Read the model definition and answer for the solid it produces. Units are mm, in the model's axes. A direction names the side the tool comes from. Give positions to 0.01 mm unless a question says otherwise; leave off trailing zeros. Loops run counter-clockwise (first coordinate to the right, second up) from the corner with the lowest first, then second, coordinate; pieces in that order, holes last. Notation, with made-up numbers: (19, -14) -> (78, -14) arc R17 ccw to (78, -2) -> close; hole circle Ø5 at (-3.75, 41). An arc over 180 degrees is marked (long way). Write each question's results on one line, items separated by ' | '. Start each with the question number.
Item 1: Each of these flat-tipped pins is pushed along its axis until it touches: P1, Ø0.7, axis at x = -4, y = -0.5, coming from the -Z side; P2, Ø5, axis at x = 0, z = 39, coming from the +Y side; P3, Ø3, axis at y = -2.5, z = 0.5, coming from the -X side. Where does it stop, or does it pass through?
Item 2: Determine the mould class of faces 1 (the flat face through (-0.1, 1.6, 35.7)), 2 (the flat face through (2, -2, -12)), 3 (the cylindrical face through (0, -2, 0)), 4 (the cylindrical face through (0, 0, 43)) for opening direction Z: +Z half, -Z half, draft (parallel to the pull), parting line (faces both ways), or undercut.
Item 3: Section B-B on x = 0 is taken. Write down the section's boundary in (y, z).
Item 4: Section C-C on z = 15 is taken. Write down the section's boundary in (x, y), and give its area (3 significant figures).
Item 5: Section A-A on y = 0 is taken. State how many separate pieces and enclosed holes the cut face has, and give its area (3 significant figures).
Item 6: Find the intervals of material crossed by line 1 (Z direction, x = 0, y = 1.5); line 2 (Y direction, x = 4, z = 38); line 3 (Z direction, x = -1.75, y = -0.75), in increasing order.
Item 7: Which of the six approach directions +Z, -Z, +X, -X, +Y, -Y give full straight-line access (tool end or side, diameter ignored) to faces 5 (the flat face through (-0.1, 1.6, -35.7)), 6 (the flat face through (-0.1, -1.6, -35.7)), 7 (the flat face through (2, -2, 12)), 8 (the flat face through (-0.1, -1.6, 35.7))?
```python
from build123d import *

# Parameters (mm, degrees)
SKETCH1_R                  = 2
SCREW_SECTION_DEPTH        = 12
SKETCH2_R                  = 3.5
BAR_SECTION_DEPTH          = 21
MOUNT_SECTION_DEPTH        = 1.6
BAR_TAPER_DEPTH            = 6
MOUNT_FILLET_R             = 0.5
MOUNT_FILLET_OF_MIRROR_2_R = 0.5


with BuildPart() as part:
    # Sketch1 → Screw Section (new body)
    with BuildSketch(Plane.XY):
        Circle(SKETCH1_R)
    screw_section = extrude(amount=SCREW_SECTION_DEPTH)

    # Sketch2 → Bar Section (add)
    with BuildSketch(Plane.XY.offset(12)):
        Circle(SKETCH2_R)
    bar_section = extrude(amount=BAR_SECTION_DEPTH)

    # Sketch3 → Mount Section (add, symmetric)
    with BuildSketch(Plane(origin=(0, 0, 0), x_dir=(1, 0, 0), z_dir=(0, 1, 0))):
        with BuildLine():
            Line((5, -33), (-5, -33))
            Line((-5, -33), (-5, -38))
            ThreePointArc((-5, -38), (0, -43), (5, -38))
            Line((5, -38), (5, -33))
        make_face()
    mount_section = extrude(amount=MOUNT_SECTION_DEPTH, both=True)

    # Sketch4 → Bar Taper (cut, symmetric)
    with BuildSketch(Plane(origin=(0, 0, 0), x_dir=(0, 0, -1), z_dir=(1, 0, 0))):
        Polygon((-28, -3.5), (-33, -1.6), (-33, -3.5), align=None)
        Polygon((-28, 3.5), (-33, 1.6), (-33, 3.5), align=None)
    bar_taper = extrude(amount=BAR_TAPER_DEPTH, both=True, mode=Mode.SUBTRACT)

    # Mount Fillet
    mount_fillet_edges = [part.edges().sort_by_distance(p)[0] for p in [
        (-5, 0, 33),
        (3.401842713, -0.823083322, 33),
        (-3.5, 0, 33),
        (5, 0, 33),
    ]]
    fillet(mount_fillet_edges, radius=MOUNT_FILLET_R)

    # Sketch6 → Ball Hole (revolve, cut)
    with BuildSketch(Plane(origin=(0, 0, 0), x_dir=(0, 0, -1), z_dir=(1, 0, 0))):
        with BuildLine():
            Line((-39.920937271, -1.6), (-38, -1.6))
            Line((-38, -1.6), (-38, 1.6))
            Line((-38, 1.6), (-39.920937271, 1.6))
            ThreePointArc((-39.920937271, 1.6), (-40.5, 0), (-39.920937271, -1.6))
        make_face()
    ball_hole = revolve(axis=Axis((0, -1.6, 38), (0, 1, 0)), mode=Mode.SUBTRACT)

    # Mirror 2: Screw Section, Bar Section, Mount Section, Bar Taper, Ball Hole across plane
    add(screw_section.mirror(Plane.XY))
    add(bar_section.mirror(Plane.XY))
    add(mount_section.mirror(Plane.XY))
    add(bar_taper.mirror(Plane.XY), mode=Mode.SUBTRACT)
    add(ball_hole.mirror(Plane.XY), mode=Mode.SUBTRACT)

    # Mount Fillet of Mirror 2
    mount_fillet_of_mirror_2_edges = [part.edges().sort_by_distance(p)[0] for p in [
        (-5, 0, -33),
        (3.401842713, -0.823083322, -33),
        (-3.5, 0, -33),
        (5, 0, -33),
    ]]
    fillet(mount_fillet_of_mirror_2_edges, radius=MOUNT_FILLET_OF_MIRROR_2_R)


solid = part.part
```
Findings:
1) P1: z = -41.42 | P2: y = 1.6 | P3: x = -1.73
2) face 1: draft | face 2: undercut | face 3: undercut | face 4: +Z half
3) outline: (-3.5, -28) -> (-1.6, -33) -> (-1.6, -36.08) arc R2.5 cw to (1.6, -36.08) -> (1.6, -33) -> (3.5, -28) -> (3.5, -12) -> (2, -12) -> (2, 12) -> (3.5, 12) -> (3.5, 28) -> (1.6, 33) -> (1.6, 36.08) arc R2.5 cw to (-1.6, 36.08) -> (-1.6, 33) -> (-3.5, 28) -> (-3.5, 12) -> (-2, 12) -> (-2, -12) -> (-3.5, -12) -> close; (-1.6, -43) -> (1.6, -43) -> (1.6, -39.92) arc R2.5 cw to (-1.6, -39.92) -> close; (-1.6, 39.92) arc R2.5 cw to (1.6, 39.92) -> (1.6, 43) -> (-1.6, 43) -> close
4) outline: circle Ø7 at (0, 0) | area: 38.5 mm2
5) separate pieces: 1 | enclosed holes: 2 | area: 529 mm2
6) line 1: -43 to -40, -36 to 36, 40 to 43 | line 2: -1.6 to 1.6 | line 3: -42.68 to -39.62, -36.38 to 36.38, 39.62 to 42.68
7) face 5: -Z, +X, -X, +Y | face 6: -Z, +X, -X, -Y | face 7: none | face 8: +Z, +X, -X, -Y
